Answer from the drawing. Dimensions are ordinates in mm from the lowest x, y and z of the part. A direction names the side the tool comes from. Coordinates: 2 decimals unless noted, no trailing zeros. Order: outer loops, then holes, each group sorted by start corner. A loop starts at its lowest first (then second) coordinate and runs counter-clockwise, first axis right, second up. Notation, with made-up numbers: M 83.25,52 L 130.25,52 A5 cw 130.25,60 Z; hole C 70,-0.5 d2. An arc over 180 degrees is marked long. Write each question's results on one line, items separated by ' | '.
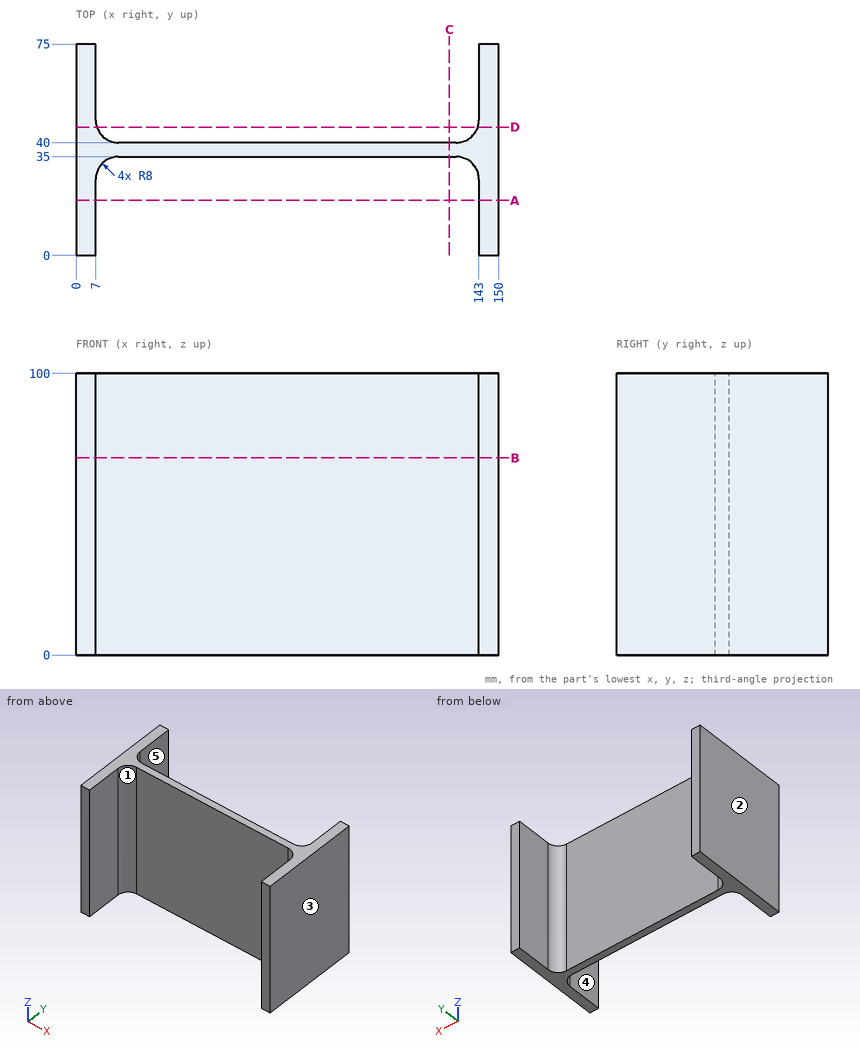
(1) The part is cut by section D-D, the plane y = 45.5. Write down the section's boundary in (x, z).
Conclusion:
outline: M 0,0 L 7.4,0 L 7.4,100 L 0,100 Z; M 142.6,0 L 150,0 L 150,100 L 142.6,100 Z
(2) Given pin 1 (3 mm diameter, centred on y = 29.5, z = 14.5, fed in from -X); pin 2 (10 mm diameter, centred on x = 116.5, z = 43.5, fed in from +Y); pin 3 (6 mm diameter, centred on x = 94, z = 39.5, fed in from -Y); pin 4 (8 mm diameter, centred on x = 117, y = 28, fed in from +Z), each flat-ended and moving along its own axis, determine where each tip first touches the part or whether it passes through.
Conclusion:
pin 1: x = 0 | pin 2: y = 40 | pin 3: y = 35 | pin 4: through
(3) The mould has two halves that part along X. Classify the marked faces 1, 2 and 3: pulls with the +X half, pulls with the -X half, needs draft (parallel to the pull), parting line crosses it, or undercut.
Conclusion:
face 1: undercut | face 2: pulls with the -X half | face 3: pulls with the +X half
(4) The part is cut by section A-A, the plane y = 19.5. Write down the section's boundary in (x, z).
Conclusion:
outline: M 0,0 L 7,0 L 7,100 L 0,100 Z; M 143,0 L 150,0 L 150,100 L 143,100 Z
(5) The part is cut by section C-C, the plane x = 132.5. Write down the section's boundary in (y, z), then the cut area to 3 significant figures.
Conclusion:
outline: M 35,0 L 40,0 L 40,100 L 35,100 Z | area: 500 mm²
(6) The part is cut by section B-B, the plane z = 70. Write down the section's boundary in (x, y).
Conclusion:
outline: M 0,0 L 7,0 L 7,27 A8 cw 15,35 L 135,35 A8 cw 143,27 L 143,0 L 150,0 L 150,75 L 143,75 L 143,48 A8 cw 135,40 L 15,40 A8 cw 7,48 L 7,75 L 0,75 Z
(7) For the marked faces 4 and 5, determine the directions among +Z, -Z, +X, -X, +Y, -Y from which every point of the face is accessible in a straight line to the end or side of a thin tool.
Conclusion:
face 4: +Z, -Z, -Y | face 5: +Z, -Z, +Y
(8) Straight lines are drawn through the part: line 1 (X direction, y = 65.5, z = 38); line 2 (Y direction, x = 21.5, z = 63); line 3 (X direction, y = 31, z = 38). For each, find the intervals that lie inside material, in ascending order.
Conclusion:
line 1: 0 to 7, 143 to 150 | line 2: 35 to 40 | line 3: 0 to 8.07, 141.93 to 150
